from build123d import *

# Parameters (mm, degrees)
F1_DEPTH = 3.048


with BuildPart() as f1:
    # F0 (on Front) → F1 (new body)
    with BuildSketch(Plane.XZ):
        with BuildLine():
            ThreePointArc((0, 19.277473), (13.631232, 13.631232), (19.277473, 0))
            ThreePointArc((19.277473, 0), (0, -19.277473), (-19.277473, 0))
            Line((-19.277473, 0), (-24.200103, -14.086255))
            Line((-24.200103, -14.086255), (-32.447593, -37.686701))
            Line((-32.447593, -37.686701), (-13.343572, -27.349228))
            Line((-13.343572, -27.349228), (0, -20.12882))
            Line((0, -20.12882), (17.126714, -25.274702))
            Line((17.126714, -25.274702), (36.677146, -31.148814))
            Line((36.677146, -31.148814), (26.117608, -11.634409))
            Line((26.117608, -11.634409), (19.822054, 0))
            Line((19.822054, 0), (23.947323, 17.233988))
            Line((23.947323, 17.233988), (28.072593, 34.467977))
            Line((28.072593, 34.467977), (11.074049, 25.269808))
            Line((11.074049, 25.269808), (0, 19.277473))
        make_face()
        with BuildLine():
            ThreePointArc((-19.277473, 0), (-13.631232, 13.631232), (0, 19.277473))
            Line((0, 19.277473), (-15.617592, 25.532357))
            Line((-15.617592, 25.532357), (-37.928615, 34.467977))
            Line((-37.928615, 34.467977), (-24.637008, 9.904611))
            Line((-24.637008, 9.904611), (-19.277473, 0))
        make_face()
        Polygon((-15.617592, 25.532357), (0, 19.277473), (11.074049, 25.269808), (11.074049, 26.854567), (0, 44.573046), align=None)
        Polygon((-24.200103, -14.086255), (-19.277473, 0), (-24.637008, 9.904611), (-45.542024, 0), align=None)
        Polygon((47.618411, 0), (23.947323, 17.233988), (19.822054, 0), (26.117608, -11.634409), align=None)
        Polygon((0, -20.12882), (-13.343572, -27.349228), (0, -52.008626), (17.126714, -25.274702), align=None)
    extrude(amount=F1_DEPTH)


solid = f1.part
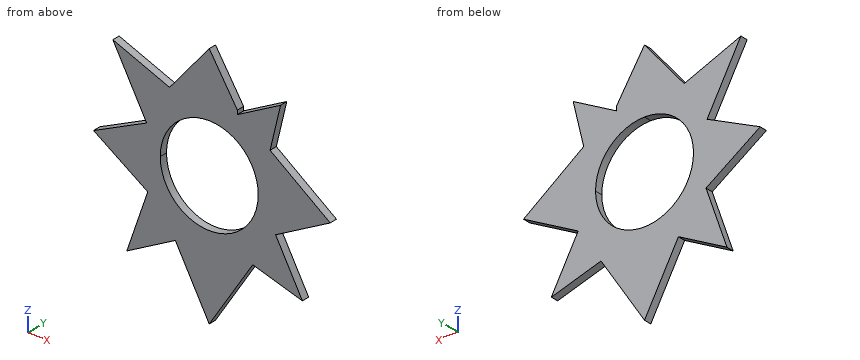
Verification items for the finished model (mm, model axes). Coordinates: 2 decimals unless noted, no trailing zeros. Order: outer loops, then holes, each group sorted by start corner. A loop starts at its lowest first (then second) coordinate and runs counter-clockwise, first axis right, second up. Notation, with made-up numbers: M -31.5,34 L 3.5,34 A20 ccw 3.5,59 Z; hole C 62.25,79 d6. An arc over 180 degrees is marked long. One line per item, written item: value. Start each with the question number.
Item 1: Sectioned sample at A-A (y = -0.75). Enter the section's corners in (x, z), then the cut area to 3 significant figures.
Item 2: Sectioned sample at D-D (x = -4). Enter the section's corners in (y, z), then the cut area to 3 significant figures.
Item 3: Sectioned sample at C-C (z = 13). Enter the section's corners in (x, y).
Item 4: Sectioned sample at B-B (x = -27). Enter the section's corners in (y, z), then the cut area to 3 significant figures.
Item 5: Scan lines: probe 1 along Z at (x, y) = (5.5, -0.25); probe 2 along Z at (x, y) = (32, -0.9); probe 3 along X at (y, z) = (-0.55, -8.5). Record each from-to range of solid material in increasing order.
Item 6: Gauge pin test, flat ends, axial feed: pin 1 (1 mm diameter, centred on y = -0.5, z = -23.5, fed in from -X); pin 2 (0.5 mm diameter, centred on y = -1, z = 25.5, fed in from +X); pin 3 (1.5 mm diameter, centred on x = 16, y = -0.5, fed in from +Z). Record the tip position at first contact, or that the pin passes through.
Conclusion:
1. outline: M -45.54,0 L -24.2,-14.09 L -32.45,-37.69 L -13.34,-27.35 L 0,-52.01 L 17.13,-25.27 L 36.68,-31.15 L 26.12,-11.63 L 47.62,0 L 23.95,17.23 L 28.07,34.47 L 11.07,25.27 L 11.07,26.85 L 0,44.57 L -15.62,25.53 L -37.93,34.47 L -24.64,9.9 Z; hole C 0,0 d38.55
1. area: 3,060 mm^2
2. outline: M -3.05,-44.62 L 0,-44.62 L 0,-18.86 L -3.05,-18.86 Z; M -3.05,18.86 L 0,18.86 L 0,39.7 L -3.05,39.7 Z
2. area: 142 mm^2
3. outline: M -26.31,-3.05 L -14.23,-3.05 L -14.23,0 L -26.31,0 Z; M 14.23,-3.05 L 29.76,-3.05 L 29.76,0 L 14.23,0 Z
4. outline: M -3.05,-34.74 L 0,-34.74 L 0,-22.1 L -3.05,-22.1 Z; M -3.05,-12.24 L 0,-12.24 L 0,8.79 L -3.05,8.79 Z; M -3.05,14.27 L 0,14.27 L 0,30.09 L -3.05,30.09 Z
4. area: 151 mm^2
5. probe 1: z = -43.42 to -18.48, 18.48 to 35.77
5. probe 2: z = -29.74 to -22.51, -8.45 to 11.37
5. probe 3: x = -32.66 to -17.3, 17.3 to 31.91
6. pin 1: stops at x = -27.66
6. pin 2: stops at x = 25.99
6. pin 3: stops at z = 28.34
